Build history of the part. All positions in model axes, mm. A direction names the side the tool comes from. Round coordinates to 2 decimals unless told otherwise and drop trailing zeros. Write each loop counter-clockwise with the first axis right and the second up, starting at its lowest first coordinate (ties: lowest second). Pieces come first, ordered by that corner, then holes. Notation, with made-up numbers: M -38,84.25 L -3,84.25 A9 cw -3,96.25 Z; hole C 58,3.25 d8. An arc over 180 degrees is marked long. Write item = value, one per line.
from build123d import *

# Parameters (mm, degrees)
FILLET1_R = 1


with BuildPart() as part:
    # Sketch1 → Revolve1 (revolve)
    with BuildSketch(Plane.XY):
        with BuildLine():
            Line((0, 0), (26.286199912, 0))
            Line((26.286199912, 0), (26.286199912, 2.410114973))
            Line((26.286199912, 2.410114973), (28.735209439, 2.410114973))
            Line((28.735209439, 2.410114973), (28.735209439, 16.726222584))
            ThreePointArc((28.735209439, 16.726222584), (19.520083074, 23.437939861), (14.857488789, 33.841108478))
            Line((14.857488789, 33.841108478), (12.063535171, 33.841108478))
            ThreePointArc((12.063535171, 33.841108478), (9.145229836, 24.235071542), (0, 20.092943721))
            Line((0, 20.092943721), (0, 0))
        make_face()
    revolve(axis=Axis((0, 0, 0), (0, 1, 0)))

    # Fillet1
    fillet1_edges = [part.edges().sort_by_distance(p)[0] for p in [
        (-28.735209439, 16.726222584, 0),
        (-26.286199912, 0, 0),
    ]]
    fillet(fillet1_edges, radius=FILLET1_R)


solid = part.part
1. Probe probe 1 along X at (y, z) = (27, 4); probe 2 along Z at (x, y) = (10.5, 29); probe 3 along X at (y, z) = (12, -5.5). List the from-to ranges inside material, lowest first.
Responses:
probe_1 = -16.69 to -10.22, 10.22 to 16.69
probe_2 = -12.37 to -5.21, 5.21 to 12.37
probe_3 = -28.2 to 28.2
2. Tool access for faces 1 (the face through (-1.2, 33.841, -12.2)), 2 (the face through (-20.86, 1.715, 15.995)): list every direction of +Z, -Z, +X, -X, +Y, -Y with a clear straight run to the whole face (end or side of a thin tool).
Responses:
face_1 = +Z, -Z, +X, -X, +Y
face_2 = -Y
3. Band-saw the part on A-A (y = 6). List the corners of the cut face in (x, z).
Responses:
outline = C 0,0 d57.47
4. Flat gauge pins, fed straight in: pin 1 (8 mm diameter, centred on x = -16, y = 22.5, fed in from +Z); pin 2 (1 mm diameter, centred on y = 11.5, z = 13, fed in from +X); pin 3 (1.5 mm diameter, centred on y = 11.5, z = 19.5, fed in from -X) (3 decimals). Where does each tip first touch, or does it go through?
Responses:
pin_1 = 19.99
pin_2 = 25.87
pin_3 = -21.775
